```python
from build123d import *

# Parameters (mm, degrees)
BOSS_EXTRUDE1_DEPTH = 7
CUT_EXTRUDE1_DEPTH  = 5
SKETCH3_R           = 3.1
CUT_EXTRUDE2_DEPTH  = 3
FILLET1_R           = 2


with BuildPart() as part:
    # Sketch1 → Boss-Extrude1 (new body)
    with BuildSketch(Plane(origin=(0, 0, 0), x_dir=(1, 0, 0), z_dir=(0, 1, 0))):
        with BuildLine():
            ThreePointArc((-8.660254038, 15), (0, 10), (8.660254038, 15))
            ThreePointArc((8.660254038, 15), (8.660254038, 5), (17.320508076, 0))
            ThreePointArc((17.320508076, 0), (8.660254038, -5), (8.660254038, -15))
            ThreePointArc((8.660254038, -15), (0, -10), (-8.660254038, -15))
            ThreePointArc((-8.660254038, -15), (-8.660254038, -5), (-17.320508076, 0))
            ThreePointArc((-17.320508076, 0), (-8.660254038, 5), (-8.660254038, 15))
        make_face()
    extrude(amount=BOSS_EXTRUDE1_DEPTH)

    # Sketch2 → Cut-Extrude1 (cut)
    with BuildSketch(Plane(origin=(0, 7, 0), x_dir=(1, 0, 0), z_dir=(0, 1, 0))):
        Polygon((0, -5.946707773), (5.15, -2.973353886), (5.15, 2.973353886), (0, 5.946707773), (-5.15, 2.973353886), (-5.15, -2.973353886), align=None)
    extrude(amount=-CUT_EXTRUDE1_DEPTH, mode=Mode.SUBTRACT)

    # Sketch3 → Cut-Extrude2 (cut, through all)
    with BuildSketch(Plane(origin=(0, 2, 0), x_dir=(1, 0, 0), z_dir=(0, 1, 0))):
        Circle(SKETCH3_R)
    extrude(amount=-CUT_EXTRUDE2_DEPTH, mode=Mode.SUBTRACT)

    # Fillet1
    fillet1_edges = [part.edges().sort_by_distance(p)[0] for p in [
        (8.660254038, 7, -5),
        (-8.660254038, 3.5, 15),
        (-17.320508076, 3.5, 0),
        (-8.660254038, 3.5, -15),
        (8.660254038, 3.5, -15),
        (17.320508076, 3.5, 0),
        (8.660254038, 3.5, 15),
        (0, 7, -10),
        (-8.660254038, 7, -5),
        (-8.660254038, 7, 5),
        (0, 7, 10),
        (-8.660254038, 0, 5),
        (-8.660254038, 0, -5),
        (0, 0, -10),
        (8.660254038, 7, 5),
        (8.660254038, 0, -5),
        (8.660254038, 0, 5),
        (0, 0, 10),
    ]]
    fillet(fillet1_edges, radius=FILLET1_R)


solid = part.part
```
Build history of the part. All positions in model axes, mm. A direction names the side the tool comes from. Round coordinates to 2 decimals unless told otherwise and drop trailing zeros.
Item 1: Drill centre lines: line 1 along Y through (x, z) = (5, 0.75); line 2 along Z through (x, y) = (3.75, 3.25); line 3 along Z through (x, y) = (-2.25, 3.75). Where is each one in solid material? Low to high.
Item 2: Pin check, flat tips, straight feed: P1, Ø2.5, axis at y = 4.5, z = 1.5, coming from the +X side; P2, Ø8, axis at x = 0, z = -1, coming from the +Y side; P3, Ø1.5, axis at x = -6, y = 6, coming from the +Z side. Stop position of each tip, or through.
Item 3: Which spindle directions (+Z, -Z, +X, -X, +Y, -Y) get a long thin tool onto all of the face, cutting with end or side? Do faces 1 (the face through (3, 0, 2)), 2 (the face through (2.54, 4.54, 4.48)). Say none if no direction does.
Item 4: Two-plate mould, pull along Z, no slides. Class faces 3 (the face through (-2.61, 4.54, 4.44)), 4 (the face through (8.628, 3.479, -5.056)), 5 (the face through (-8.628, 3.479, 5.056)): released by +Z, released by -Z, zero draft, split by the parting line, or undercut.
Worked answers:
1. line 1: y = 0 to 2
1. line 2: z = -10.73 to -3.78, 3.78 to 10.73
1. line 3: z = -10.26 to -4.65, 4.65 to 10.26
2. P1: stops at x = 12.67
2. P2: stops at y = 2
2. P3: stops at z = 11.21
3. face 1: +Z, -Z, +X, -X, -Y
3. face 2: +Y
4. face 3: undercut
4. face 4: released by -Z
4. face 5: released by +Z
